from build123d import *

# Parameters (mm, degrees)
F5_W     = 4.1
F5_H     = 2.55
F5_W_2   = 3.1
F5_H_2   = 1.55
F5_R     = 9.525
F7_DEPTH = 6.35
F0_R     = 9.525
F0_W     = 2.55
F0_H     = 4.1
F8_DEPTH = 6.35


with BuildPart() as f6:
    # F6: sweep along a path in F3, F1
    with BuildLine(Plane.XZ.offset(262.4)) as f6_path:
        Line((150.8, -25.4), (150.8, -15.4))
        ThreePointArc((150.8, -15.4), (146.2894444303, -4.5105555697), (135.4, 0))
        Line((135.4, 0), (125.4, 0))
    with BuildLine(Plane.XY) as f6_path_2:
        Line((125.4, -262.4), (25.4, -262.4))
        Line((25.4, -262.4), (15.4, -262.4))
        ThreePointArc((15.4, -262.4), (4.5105555697, -257.8894444303), (0, -247))
        Line((0, -247), (0, -237))
        Line((0, -237), (0, 0))
    # F5 (on offset) → F6 (sweep)
    with BuildSketch(Plane.XY.offset(-25.4)):
        with Locations((150.8, -262.4)):
            Rectangle(F5_W, F5_H)
        with Locations((150.8, -262.4)):
            Rectangle(F5_W_2, F5_H_2, mode=Mode.SUBTRACT)
    sweep(path=f6_path.line + f6_path_2.line)

    # F5 (on offset) → F7 (join)
    with BuildSketch(Plane.XY.offset(-25.4)):
        with Locations((150.8, -262.4)):
            Circle(F5_R)
        with Locations((150.8, -262.4)):
            Rectangle(F5_W, F5_H, mode=Mode.SUBTRACT)
    extrude(amount=F7_DEPTH)

    # F0 (on Front) → F8 (join)
    with BuildSketch(Plane.XZ):
        Circle(F0_R)
        Rectangle(F0_W, F0_H, mode=Mode.SUBTRACT)
    extrude(amount=F8_DEPTH)


solid = f6.part
Part model, mm, in its own coordinate system. A direction names the side the tool comes from. Give positions to 0.01 mm unless a question says otherwise; leave off trailing zeros. Loops run counter-clockwise (first coordinate to the right, second up) from the corner with the lowest first, then second, coordinate; pieces in that order, holes last. Notation, with made-up numbers: (49.25, 59.25) -> (88.25, 59.25) arc R29 ccw to (88.25, 89.25) -> close; hole circle Ø9 at (-13.5, -34). An arc over 180 degrees is marked (long way). Write each question's results on one line, items separated by ' | '. Start each with the question number.
Q1. Pull direction Z, two halves, no side cores. Call faces 4 (the face through (90, -261.125, -1)), 5 (the face through (147.52, -262.41, -3.55)), 6 (the face through (145.301, -262.389, -5.715)), 7 (the face through (153, -262, -25.4)): +Z half, -Z half, draft (parallel to the pull), parting line (faces both ways), or undercut.
Q2. Wall check: L1, parallel to Y at x = 124, z = -1 (3 decimals); L2, parallel to X at y = -152, z = -0.5 (3 decimals); L3, parallel to Y at x = 8.5, z = 3. Give the ranges that are in metal, low to high.
Q3. Pin check, flat tips, straight feed: P1, Ø1.2, axis at y = -262.5, z = -18, coming from the +X side; P2, Ø3.5, axis at y = -138, z = 0, coming from the +X side (3 decimals); P3, Ø1.3, axis at y = -262.5, z = -17, coming from the -X side. Stop position of each tip, or through.
Q4. Band-saw the part on B-B on y = -199.5. List the corners of the cut face in (x, z) (3 decimals), plus the area to 3 significant figures.
Q5. Which spindle directions (+Z, -Z, +X, -X, +Y, -Y) get a long thin tool onto all of the face, cutting with end or side? Do faces 1 (the face through (89, -263.675, -1)), 2 (the face through (144.94, -262.42, -6.06)), 3 (the face through (94, -261.625, -1)). Say none if no direction does.
Q6. Band-saw the part on A-A on x = 5. List the corners of the cut face in (y, z).
Q7. Band-saw the part on C-C on x = 103. List the corners of the cut face in (y, z) (3 decimals), plus the area to 3 significant figures.
Results are:
1) face 4: draft | face 5: undercut | face 6: undercut | face 7: -Z half
2) L1: y = -263.675 to -263.175, -261.625 to -261.125 | L2: x = -1.275 to -0.775, 0.775 to 1.275 | L3: y = -6.35 to 0
3) P1: stops at x = 152.85 | P2: stops at x = 1.275 | P3: stops at x = 148.75
4) outline: (-1.275, -2.05) -> (1.275, -2.05) -> (1.275, 2.05) -> (-1.275, 2.05) -> close; hole (-0.775, -1.55) -> (0.775, -1.55) -> (0.775, 1.55) -> (-0.775, 1.55) -> close | area: 5.65 mm²
5) face 1: +Z, +X, -X, -Y | face 2: -X, +Y, -Y | face 3: none
6) outline: (-260.03, -2.05) -> (-256.56, -2.05) -> (-256.56, 2.05) -> (-260.03, 2.05) -> close; (-6.35, -8.11) -> (0, -8.11) -> (0, 8.11) -> (-6.35, 8.11) -> close; hole (-259.39, -1.55) -> (-257.28, -1.55) -> (-257.28, 1.55) -> (-259.39, 1.55) -> close
7) outline: (-263.675, -2.05) -> (-261.125, -2.05) -> (-261.125, 2.05) -> (-263.675, 2.05) -> close; hole (-263.175, -1.55) -> (-261.625, -1.55) -> (-261.625, 1.55) -> (-263.175, 1.55) -> close | area: 5.65 mm²
